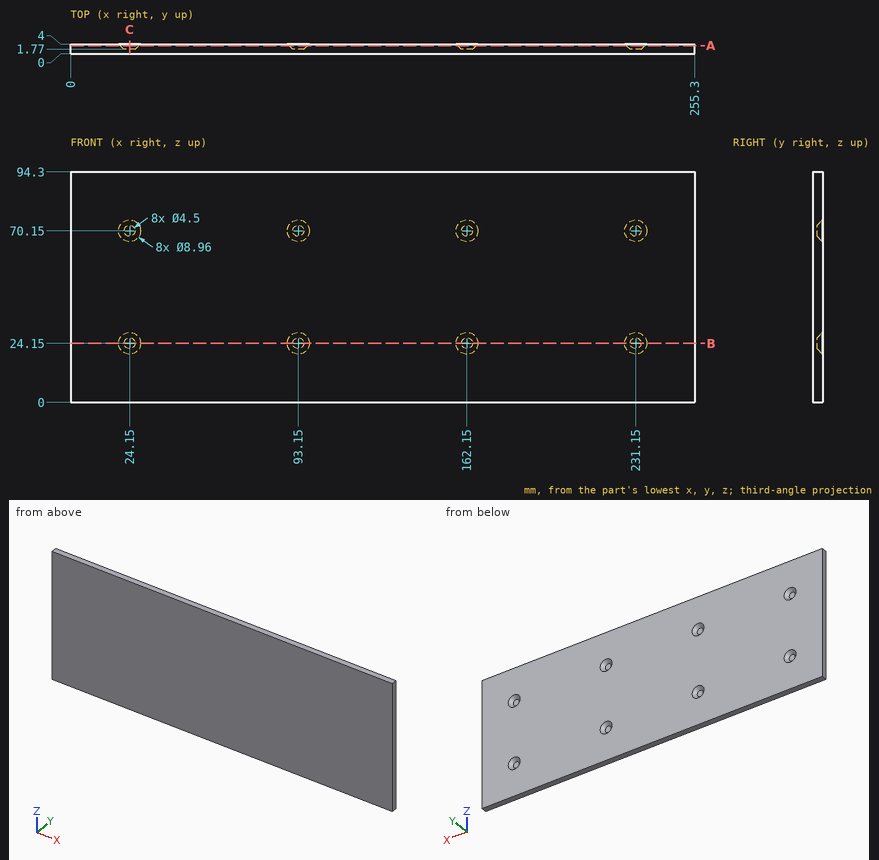
Print and shaded views of the part. All mm, measured from the part's lowest x, y and z. Coordinates: 2 decimals unless noted, no trailing zeros. Write each loop counter-clockwise with the first axis right and the second up, starting at its lowest first coordinate (ties: lowest second). Pieces come first, ordered by that corner, then holes.
(1) Cut at B-B, the plane z = 24.15. List the corners of the cut face in (x, y).
(2) Flat gauge pins, fed straight in: pin 1 (4 mm diameter, centred on x = 58, z = 75.5, fed in from -Y); pin 2 (5 mm diameter, centred on x = 161.5, z = 23.5, fed in from +Y); pin 3 (3.5 mm diameter, centred on x = 93, z = 24.5, fed in from +Y). Where does each tip first touch, or does it go through?
(3) Cut at A-A, the plane y = 3.35. Count the separate pieces of the cut face and the enclosed holes in it, and give its area (3 significant figures).
(4) Cut at C-C, the plane x = 24.15. List the corners of the cut face in (y, z), and give its area (3 significant figures).
(5) Drill centre lines: probe 1 along X at (y, z) = (2.7, 26); probe 2 along Y at (x, z) = (231, 71.5). Where is each one in solid material? Low to high.
Geometry says:
1. outline: (0, 0) - (255.3, 0) - (255.3, 4) - (235.63, 4) - (233.4, 1.77) - (228.9, 1.77) - (226.67, 4) - (166.63, 4) - (164.4, 1.77) - (159.9, 1.77) - (157.67, 4) - (97.63, 4) - (95.4, 1.77) - (90.9, 1.77) - (88.67, 4) - (28.63, 4) - (26.4, 1.77) - (21.9, 1.77) - (19.67, 4) - (0, 4) - close
2. pin 1: stops at y = 0
2. pin 2: stops at y = 2.94
2. pin 3: stops at y = 1.77
3. separate pieces: 1
3. enclosed holes: 8
3. area: 23,700 mm2
4. outline: (0, 0) - (4, 0) - (4, 19.67) - (1.77, 21.9) - (1.77, 26.4) - (4, 28.63) - (4, 65.67) - (1.77, 67.9) - (1.77, 72.4) - (4, 74.63) - (4, 94.3) - (0, 94.3) - close
4. area: 347 mm2
5. probe 1: x = 0 to 21.56, 26.74 to 90.56, 95.74 to 159.56, 164.74 to 228.56, 233.74 to 255.3
5. probe 2: y = 0 to 1.77
